Input: dimensioned drawing with shaded views. Units: mm. Origin: part minimum x, y, z. Coordinates: 2 decimals unless noted, no trailing zeros. Loops run counter-clockwise (first coordinate to the right, second up) from the corner with the lowest first, then second, coordinate; pieces in that order, holes last.
(1) Section B-B, the plane y = 9.75. Return loops of the section in (x, z).
(2) Line query: L1, parallel to X at y = 9, z = 0.1; L2, parallel to Y at x = 71.5, z = 0.6; L3, parallel to Y at x = 32, z = 0.75. Output: solid intervals per line, ascending.
(3) Section A-A, the plane x = 39.5. Return loops of the section in (y, z), then the cut area to 3 significant figures.
(4) Section D-D, the plane y = 13. Return loops of the section in (x, z), then the cut area to 3 significant figures.
(5) Contact query for a flat-ended pin moving along its axis: P1, Ø0.5, axis at y = 10, z = 0.5, coming from the -X side. Output: stop coordinate, or through.
(6) Section C-C, the plane z = 0.4. Return loops of the section in (x, y), then the cut area to 3 significant figures.
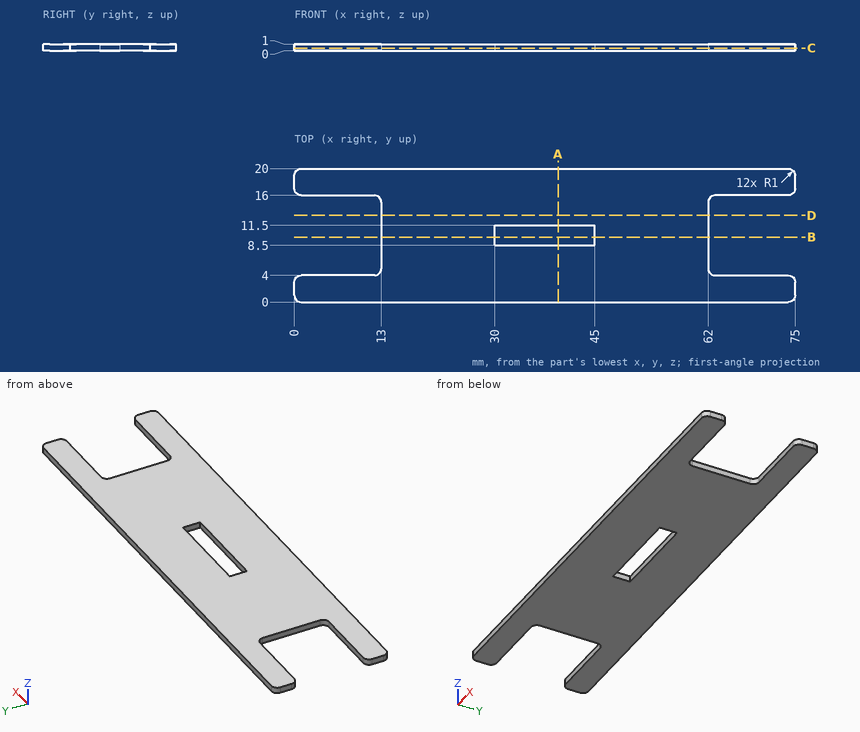
Report:
1. outline: (13, 0) - (30, 0) - (30, 1) - (13, 1) - close; (45, 0) - (62, 0) - (62, 1) - (45, 1) - close
2. L1: x = 13 to 30, 45 to 62
2. L2: y = 0 to 4, 16 to 20
2. L3: y = 0 to 8.5, 11.5 to 20
3. outline: (0, 0) - (8.5, 0) - (8.5, 1) - (0, 1) - close; (11.5, 0) - (20, 0) - (20, 1) - (11.5, 1) - close
3. area: 17.0 mm2
4. outline: (13, 0) - (62, 0) - (62, 1) - (13, 1) - close
4. area: 49.0 mm2
5. P1: stops at x = 13
6. outline: (0, 1) arc R1 ccw to (1, 0) - (74, 0) arc R1 ccw to (75, 1) - (75, 3) arc R1 ccw to (74, 4) - (63, 4) arc R1 cw to (62, 5) - (62, 15) arc R1 cw to (63, 16) - (74, 16) arc R1 ccw to (75, 17) - (75, 19) arc R1 ccw to (74, 20) - (1, 20) arc R1 ccw to (0, 19) - (0, 17) arc R1 ccw to (1, 16) - (12, 16) arc R1 cw to (13, 15) - (13, 5) arc R1 cw to (12, 4) - (1, 4) arc R1 ccw to (0, 3) - close; hole (30, 8.5) - (45, 8.5) - (45, 11.5) - (30, 11.5) - close
6. area: 1,140 mm2
